Source: CAD feature listing. Evaluate the final solid. Frame: model axes, mm. Round coordinates to 2 decimals unless told otherwise and drop trailing zeros. Order: outer loops, then holes, each group sorted by start corner. A loop starts at its lowest first (then second) coordinate and runs counter-clockwise, first axis right, second up. Notation, with made-up numbers: (61.5, 69.25) -> (100.5, 69.25) arc R29 ccw to (100.5, 94.25) -> close; hole circle Ø3 at (48.25, -34.5). An arc over 180 degrees is marked (long way). Use a Markdown table: item, result. Add a question column.
```python
from build123d import *

# Parameters (mm, degrees)
F0_R     = 9.525
F0_R_2   = 4.7625
F1_DEPTH = 16.51


with BuildPart() as f1:
    # F0 (on Top) → F1 (new body)
    with BuildSketch(Plane.XY):
        with BuildLine():
            ThreePointArc((-12.591503, 1.656522), (-0.830035, -12.672847), (12.7, 0))
            ThreePointArc((12.7, 0), (12.672847, 0.830036), (12.591503, 1.656522))
            ThreePointArc((12.591503, 1.656522), (0, 12.7), (-12.591503, 1.656522))
        make_face()
        Circle(F0_R, mode=Mode.SUBTRACT)
        with BuildLine():
            ThreePointArc((-12.591503, 1.656522), (0, 12.7), (12.591503, 1.656522))
            Line((12.591503, 1.656522), (7.869689, 37.547826))
            ThreePointArc((7.869689, 37.547826), (7.920529, 37.031272), (7.9375, 36.5125))
            ThreePointArc((7.9375, 36.5125), (-0.518772, 28.591971), (-7.869689, 37.547826))
            Line((-7.869689, 37.547826), (-12.591503, 1.656522))
        make_face()
        with BuildLine():
            ThreePointArc((7.9375, 36.5125), (7.920529, 37.031272), (7.869689, 37.547826))
            ThreePointArc((7.869689, 37.547826), (0, 44.45), (-7.869689, 37.547826))
            ThreePointArc((-7.869689, 37.547826), (-0.518772, 28.591971), (7.9375, 36.5125))
        make_face()
        with Locations((0, 36.5125)):
            Circle(F0_R_2, mode=Mode.SUBTRACT)
    extrude(amount=F1_DEPTH)


solid = f1.part
```
1) Draft query along X for faces 1 (the cylindrical face through (12.674, 0.818, 8.139)), 2 (the flat face through (-10.2, 19.85, 8.14)), 3 (the cylindrical face through (-7.559, -5.796, 8.139)), 4 (the cylindrical face through (-1.032, 31.863, 8.139)). Return one class per face: pulls with the +X half, pulls with the -X half, needs draft (parallel to the pull), parting line crosses it, or undercut.
2) Section A-A on x = 0. Output: boundary loops of the cut face in (y, z) (3 decimals).
3) Section C-C on z = 15.5. Count the separate pieces of the cut face and the enclosed holes in it, then the cut area to 3 significant figures.
4) Section B-B on y = 34. Output: boundary loops of the cut face in (x, z), then the cut area to 3 significant figures.
5) First-contact query: pin 1 Ø5 at (y, z) = (36, 2.5) entering from -X; pin 2 Ø3 at (y, z) = (8.5, 5.5) entering from +X; pin 3 Ø8 at (y, z) = (36, 10) entering from +X; pin 4 Ø1 at (x, y) = (-5, 10.5) entering from -Z. Flat tips, straight axial feed; report the tip coordinate or a pass-through.
6) Section D-D on x = -2.75. Output: boundary loops of the cut face in (y, z), then the cut area to 3 significant figures.
7) Line query: probe 1 along X at (y, z) = (39, 12); probe 2 along Y at (x, z) = (-1.75, 9.5); probe 3 along X at (y, z) = (38, 12.25). Output: solid intervals per line, ascending. Write a range as from..to.
Conclusion:
| question | item | result |
|---|---|---|
| 1 | face 1 | pulls with the +X half |
| 1 | face 2 | pulls with the -X half |
| 1 | face 3 | undercut |
| 1 | face 4 | undercut |
| 2 | outline | (-12.7, 0) -> (-9.525, 0) -> (-9.525, 16.51) -> (-12.7, 16.51) -> close; (9.525, 0) -> (31.75, 0) -> (31.75, 16.51) -> (9.525, 16.51) -> close; (41.275, 0) -> (44.45, 0) -> (44.45, 16.51) -> (41.275, 16.51) -> close |
| 3 | separate pieces | 1 |
| 3 | enclosed holes | 2 |
| 3 | area | 756 mm^2 |
| 4 | outline | (-8.34, 0) -> (-4.05, 0) -> (-4.05, 16.51) -> (-8.34, 16.51) -> close; (4.05, 0) -> (8.34, 0) -> (8.34, 16.51) -> (4.05, 16.51) -> close |
| 4 | area | 142 mm^2 |
| 5 | pin 1 | stops at x = -8.4 |
| 5 | pin 2 | stops at x = 11.89 |
| 5 | pin 3 | stops at x = 8.6 |
| 5 | pin 4 | stops at z = 0 |
| 6 | outline | (-12.4, 0) -> (-9.12, 0) -> (-9.12, 16.51) -> (-12.4, 16.51) -> close; (9.12, 0) -> (32.62, 0) -> (32.62, 16.51) -> (9.12, 16.51) -> close; (40.4, 0) -> (43.96, 0) -> (43.96, 16.51) -> (40.4, 16.51) -> close |
| 6 | area | 501 mm^2 |
| 7 | probe 1 | x = -7.54..-4.06, 4.06..7.54 |
| 7 | probe 2 | y = -12.58..-9.36, 9.36..32.08, 40.94..44.25 |
| 7 | probe 3 | x = -7.8..-4.52, 4.52..7.8 |
